from build123d import *

# Parameters (mm, degrees)
SKETCH4_W                       = 73.025
SKETCH4_H                       = 73.025
BOSS_EXTRUDE1_DEPTH             = 9.525
SKETCH7_R                       = 34.925
BOSS_EXTRUDE3_DEPTH             = 12.7
FILLET1_R                       = 7.9502
SKETCH8_R                       = 12.6365
BOSS_EXTRUDE4_DEPTH             = 1.6002
SKETCH9_R                       = 5.4991
BOSS_EXTRUDE5_DEPTH             = 0.7874
CUT_EXTRUDE1_START              = -12.7
CUT_EXTRUDE1_DEPTH              = 12.7
CIRPATTERN1_COUNT               = 2
SKETCH11_R                      = 5.08
CUT_EXTRUDE2_DEPTH              = 54.795548015
F_1_4_0_25_DIAMETER_HOLE1_D     = 6.35
F_1_4_0_25_DIAMETER_HOLE2_D     = 6.35
F_1_4_0_25_DIAMETER_HOLE2_DEPTH = 14.3002
F_1_4_0_25_DIAMETER_HOLE2_TIP   = 1.907732465
F_3_8_16_TAPPED_HOLE1_D         = 7.9375
F_3_8_16_TAPPED_HOLE1_DEPTH     = 15.875
F_3_8_16_TAPPED_HOLE1_TIP       = 2.384665582
CUT_EXTRUDE3_DEPTH              = 0.254


with BuildPart() as part:
    # Sketch4 → Boss-Extrude1 (new body)
    with BuildSketch(Plane(origin=(0, 0, 0), x_dir=(1, 0, 0), z_dir=(0, 1, 0))):
        Rectangle(SKETCH4_W, SKETCH4_H)
    extrude(amount=BOSS_EXTRUDE1_DEPTH)

    # Sketch7 → Boss-Extrude3 (add)
    with BuildSketch(Plane(origin=(0, 9.525, 0), x_dir=(1, 0, 0), z_dir=(0, 1, 0))):
        with Locations(Location((0, 0, 0), (0, 0, 270))):
            Circle(SKETCH7_R)
    extrude(amount=BOSS_EXTRUDE3_DEPTH)

    # Fillet1
    fillet1_edges = [part.edges().sort_by_distance(p)[0] for p in [
        (36.5125, 4.7625, 36.5125),
        (-36.5125, 4.7625, 36.5125),
        (-36.5125, 4.7625, -36.5125),
        (36.5125, 4.7625, -36.5125),
    ]]
    fillet(fillet1_edges, radius=FILLET1_R)

    # Sketch8 → Boss-Extrude4 (add)
    with BuildSketch(Plane(origin=(0, 22.225, 0), x_dir=(1, 0, 0), z_dir=(0, 1, 0))):
        with Locations(Location((0, 0, 0), (0, 0, 270))):
            Circle(SKETCH8_R)
    extrude(amount=BOSS_EXTRUDE4_DEPTH)

    # Sketch9 → Boss-Extrude5 (add)
    with BuildSketch(Plane(origin=(0, 23.8252, 0), x_dir=(1, 0, 0), z_dir=(0, 1, 0))):
        with Locations(Location((0, 0, 0), (0, 0, 270))):
            Circle(SKETCH9_R)
    extrude(amount=BOSS_EXTRUDE5_DEPTH)

    # Sketch10 → Cut-Extrude1 (cut)
    with BuildSketch(Plane(origin=(0, 22.225, 0), x_dir=(1, 0, 0), z_dir=(0, 1, 0)).offset(CUT_EXTRUDE1_START)):
        with BuildLine():
            Line((26.096624288, 14.314528257), (29.873820286, 18.091724255))
            ThreePointArc((29.873820286, 18.091724255), (24.695704333, 24.695704333), (18.091724255, 29.873820286))
            Line((18.091724255, 29.873820286), (14.314528257, 26.096624288))
            ThreePointArc((14.314528257, 26.096624288), (14.314528257, 14.314528257), (26.096624288, 14.314528257))
        make_face()
    cut_extrude1 = extrude(amount=CUT_EXTRUDE1_DEPTH, mode=Mode.SUBTRACT)

    # CirPattern1: Cut-Extrude1 ×2 about axis
    cirpattern1_axis = Axis((0, 0, 0), (0, 1, 0))
    for i in range(1, CIRPATTERN1_COUNT):
        add(cut_extrude1.rotate(cirpattern1_axis, i * 360 / CIRPATTERN1_COUNT), mode=Mode.SUBTRACT)

    # Sketch11 → Cut-Extrude2 (cut, through all)
    with BuildSketch(Plane(origin=(0, 9.525, 0), x_dir=(1, 0, 0), z_dir=(0, 1, 0))):
        with Locations(Location((20.205576272, 20.205576272, 0), (0, 0, 270))):
            Circle(SKETCH11_R)
        with Locations(Location((-20.205576272, -20.205576272, 0), (0, 0, 270))):
            Circle(SKETCH11_R)
    extrude(amount=-CUT_EXTRUDE2_DEPTH, mode=Mode.SUBTRACT)

    # 1/4 (0.25) Diameter Hole1 (through all)
    with Locations(Plane(origin=(0, 9.525, 0), x_dir=(1, 0, 0), z_dir=(0, 1, 0))):
        with Locations((-28.5623, 28.5623), (28.5623, -28.5623)):
            Hole(F_1_4_0_25_DIAMETER_HOLE1_D / 2)

    # 1/4 (0.25) Diameter Hole2
    with Locations(Plane(origin=(0, 22.225, 0), x_dir=(1, 0, 0), z_dir=(0, 1, 0))):
        with Locations((0, 25.4)):
            Hole(F_1_4_0_25_DIAMETER_HOLE2_D / 2, depth=F_1_4_0_25_DIAMETER_HOLE2_DEPTH)
            with Locations((0, 0, -(F_1_4_0_25_DIAMETER_HOLE2_DEPTH + F_1_4_0_25_DIAMETER_HOLE2_TIP / 2))):  # 118° drill point
                Cone(0, F_1_4_0_25_DIAMETER_HOLE2_D / 2, F_1_4_0_25_DIAMETER_HOLE2_TIP, mode=Mode.SUBTRACT)

    # 3/8-16 Tapped Hole1
    with Locations(Plane(origin=(0, 24.6126, 0), x_dir=(1, 0, 0), z_dir=(0, 1, 0))):
        with Locations((0, 0)):
            Hole(F_3_8_16_TAPPED_HOLE1_D / 2, depth=F_3_8_16_TAPPED_HOLE1_DEPTH)
            with Locations((0, 0, -(F_3_8_16_TAPPED_HOLE1_DEPTH + F_3_8_16_TAPPED_HOLE1_TIP / 2))):  # 118° drill point
                Cone(0, F_3_8_16_TAPPED_HOLE1_D / 2, F_3_8_16_TAPPED_HOLE1_TIP, mode=Mode.SUBTRACT)

    # Sketch18 → Cut-Extrude3 (cut)
    with BuildSketch(Plane(origin=(0, 22.225, 0), x_dir=(1, 0, 0), z_dir=(0, 1, 0))):
        Polygon((0, -28.845315502), (4.7625, -22.495315502), (1.5875, -22.495315502), (1.5875, -16.145315502), (-1.5875, -16.145315502), (-1.5875, -22.495315502), (-4.7625, -22.495315502), align=None)
    extrude(amount=-CUT_EXTRUDE3_DEPTH, mode=Mode.SUBTRACT)


solid = part.part
Source: CAD feature listing. Evaluate the final solid. Frame: model axes, mm. A direction names the side the tool comes from. Give positions to 0.01 mm unless a question says otherwise; leave off trailing zeros. Loops run counter-clockwise (first coordinate to the right, second up) from the corner with the lowest first, then second, coordinate; pieces in that order, holes last. Notation, with made-up numbers: (-19, 49) -> (14, 49) arc R24 ccw to (14, 64) -> close; hole circle Ø8 at (44, 2). An arc over 180 degrees is marked (long way). Use a Markdown table: item, result. Add a question column.
1) Reachability of faces 5 (the face through (-4, 24.613, 2)), 6 (the face through (-4.84, 23.014, 11.673)), 7 (the face through (16.23, 15.79, -28.01)) from +Z, -Z, +X, -X, +Y, -Y: full face, straight path, thin tool, end or side. Return the list, or none.
2) Section query B-B, the plane z = -7. Return the cut outline in (x, y) (1 decimal).
3) Pull-direction query (Z, two-part tool) for faces 1 (the face through (36.512, 5, 0)), 2 (the face through (-16.772, 4.829, 16.461)), 3 (the face through (0, 5, 36.512)), 4 (the face through (0, 21.971, 22)); classes: +Z half, -Z half, draft (parallel to the pull), parting line (faces both ways), or undercut.
4) First-contact query: pin 1 (5 mm diameter, centred on x = 0, z = -25.4, fed in from -Y); pin 2 (7.5 mm diameter, centred on x = -28.56, z = -28.56, fed in from +Y) (3 decimals); pin 3 (10 mm diameter, centred on y = 20, z = -23.5, fed in from +X); pin 4 (10 mm diameter, centred on y = 20.5, z = 15, fed in from -X). Flat tips, straight axial feed; report the tip coordinate or a pass-through.
5) Line query: line 1 along Z through (x, y) = (0, 19.25) (3 decimals); line 2 along X through (y, z) = (3.25, -20); line 3 along Y through (x, z) = (33.5, -3.5) (3 decimals). Output: solid intervals per line, ascending. Write a range as [from, to].
6) Section query A-A, the plane x = 16. Return the cut outline in (y, z) (1 decimal), then the cut area to 3 significant figures.
Numbers:
| question | item | result |
|---|---|---|
| 1 | face 5 | +Z, -Z, +X, -X, +Y |
| 1 | face 6 | +Y |
| 1 | face 7 | +X, +Y |
| 2 | outline | (-36.5, 0) -> (36.5, 0) -> (36.5, 9.5) -> (34.2, 9.5) -> (34.2, 22.2) -> (10.5, 22.2) -> (10.5, 23.8) -> (-10.5, 23.8) -> (-10.5, 22.2) -> (-34.2, 22.2) -> (-34.2, 9.5) -> (-36.5, 9.5) -> close |
| 3 | face 1 | draft |
| 3 | face 2 | undercut |
| 3 | face 3 | +Z half |
| 3 | face 4 | undercut |
| 4 | pin 1 | stops at y = 0 |
| 4 | pin 2 | stops at y = 9.525 |
| 4 | pin 3 | stops at x = 16.72 |
| 4 | pin 4 | stops at x = -33.46 |
| 5 | line 1 | z = [-34.925, -28.575], [-22.225, -3.969], [3.969, 34.925] |
| 5 | line 2 | x = [-36.51, 15.13], [25.28, 36.51] |
| 5 | line 3 | y = [0, 22.225] |
| 6 | outline | (0, -36.5) -> (9.5, -36.5) -> (9.5, -31) -> (22.2, -31) -> (22.2, -27.8) -> (9.5, -27.8) -> (9.5, -23.1) -> (0, -23.1) -> close; (0, -17.4) -> (9.5, -17.4) -> (9.5, -13) -> (22.2, -13) -> (22.2, 31) -> (9.5, 31) -> (9.5, 36.5) -> (0, 36.5) -> close |
| 6 | area | 1,240 mm2 |
